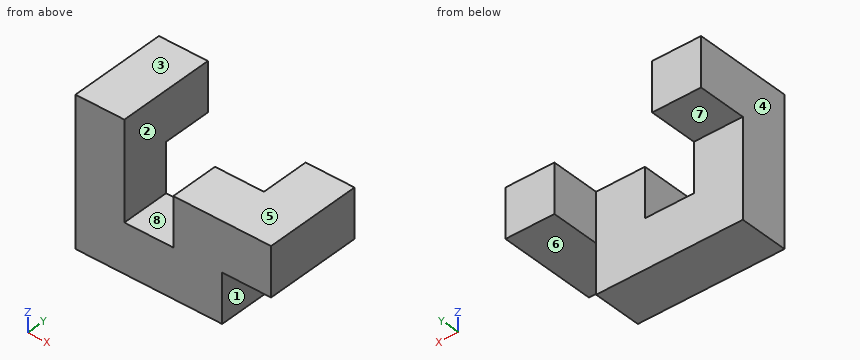
```python
from build123d import *

# Parameters (mm, degrees)
F0_W     = 12.7
F0_H     = 12.7
F1_DEPTH = 12.7
F2_DEPTH = 12.7


with BuildPart() as f1:
    # F0 (on Front) → F1 (new body)
    with BuildSketch(Plane.XZ):
        with Locations((-54.735524, 43.792849)):
            Rectangle(F0_W, F0_H)
        with Locations((-54.735524, 31.092849)):
            Rectangle(F0_W, F0_H)
        with Locations((-29.335524, 31.092849)):
            Rectangle(F0_W, F0_H)
        with Locations((-42.035524, 31.092849)):
            Rectangle(F0_W, F0_H)
        with Locations((-29.335524, 43.792849)):
            Rectangle(F0_W, F0_H)
    extrude(amount=F1_DEPTH)

    # F0 (on Front) → F2 (join, symmetric)
    with BuildSketch(Plane.XZ):
        with Locations((-54.735524, 56.492849)):
            Rectangle(F0_W, F0_H)
        with Locations((-16.635524, 43.792849)):
            Rectangle(F0_W, F0_H)
    extrude(amount=F2_DEPTH, both=True)


solid = f1.part
```
Geometry check sheet. Reference: the model listing, model coordinates, mm. Face numbers are marked on the shaded views. A direction names the side the tool comes from. Coordinates: 2 decimals unless noted, no trailing zeros. Order: outer loops, then holes, each group sorted by start corner. A loop starts at its lowest first (then second) coordinate and runs counter-clockwise, first axis right, second up. Notation, with made-up numbers: (53.25, 45.5) - (108.25, 45.5) arc R32 cw to (108.25, 73.5) - close; hole circle Ø8 at (61, -8.75). An arc over 180 degrees is marked (long way). Answer as a JSON object with one key per item and string values. Group by question number.
Item 1: Tool access check on the marked faces 5, 6, 7 and 8. Record the directions out of +Z, -Z, +X, -X, +Y, -Y that give a thin tool (end or side, any length) a straight path to the whole face; none if there is none.
Item 2: Draft check along X on the marked faces 1, 2, 3 and 4. Enter one of: +X half, -X half, draft (parallel to the pull), parting line (faces both ways), or undercut.
Item 3: Depth check by flat-ended pin: pin 1 Ø6.5 at (x, y) = (-52, 7.5) entering from -Z; pin 2 Ø5 at (x, y) = (-42, 4.5) entering from -Z; pin 3 Ø7.5 at (x, z) = (-45.5, 42.5) entering from +Y; pin 4 Ø10 at (x, y) = (-42, -5.5) entering from +Z. Enter the tip coordinate at first touch or a pass-through.
Item 4: Sectioned sample at B-B, the plane y = 10.75. Record the cut outline in (x, z).
Item 5: Sectioned sample at C-C, the plane x = -49.5. Record the cut outline in (y, z).
Item 6: Sectioned sample at D-D, the plane y = -4. Record the cut outline in (x, z), and give its area (3 significant figures).
Item 7: Sectioned sample at A-A, the plane z = 40. Record the cut outline in (x, y), and give its area (3 significant figures).
Item 8: Scan lines: probe 1 along X at (y, z) = (-8.25, 37.5); probe 2 along X at (y, z) = (-2.25, 32); probe 3 along X at (y, z) = (-10.5, 51). Record each from-to range of solid material in increasing order.
Resolved:
{
 "1": {"face 5": "+Z, +X, +Y, -Y", "face 6": "-Z, +X, +Y, -Y", "face 7": "-Z, -X, +Y", "face 8": "+Z, +Y, -Y"},
 "2": {"face 1": "+X half", "face 2": "undercut", "face 3": "draft", "face 4": "-X half"},
 "3": {"pin 1": "z = 50.14", "pin 2": "through", "pin 3": "y = 0", "pin 4": "z = 37.44"},
 "4": {"outline": "(-61.09, 50.14) - (-48.39, 50.14) - (-48.39, 62.84) - (-61.09, 62.84) - close; (-22.99, 37.44) - (-10.29, 37.44) - (-10.29, 50.14) - (-22.99, 50.14) - close"},
 "5": {"outline": "(-12.7, 24.74) - (0, 24.74) - (0, 50.14) - (12.7, 50.14) - (12.7, 62.84) - (-12.7, 62.84) - close"},
 "6": {"outline": "(-61.09, 24.74) - (-22.99, 24.74) - (-22.99, 37.44) - (-10.29, 37.44) - (-10.29, 50.14) - (-35.69, 50.14) - (-35.69, 37.44) - (-48.39, 37.44) - (-48.39, 62.84) - (-61.09, 62.84) - close", "area": "1,130 mm^2"},
 "7": {"outline": "(-61.09, -12.7) - (-48.39, -12.7) - (-48.39, 0) - (-61.09, 0) - close; (-35.69, -12.7) - (-10.29, -12.7) - (-10.29, 12.7) - (-22.99, 12.7) - (-22.99, 0) - (-35.69, 0) - close", "area": "645 mm^2"},
 "8": {"probe 1": "-61.09 to -48.39, -35.69 to -10.29", "probe 2": "-61.09 to -22.99", "probe 3": "-61.09 to -48.39"}
}
